Input: part model. Units: mm. Frame: model coordinates. A direction names the side the tool comes from. Give positions to 0.01 mm unless a question says otherwise; leave off trailing zeros. Use a Markdown table: item, result.
from build123d import *

# Parameters (mm, degrees)
SKETCH3_R           = 3.81
CUT_EXTRUDE1_DEPTH  = 51.8
SKETCH5_R           = 10.593705
SKETCH5_R_2         = 8.763
BOSS_EXTRUDE7_DEPTH = 17.78
SKETCH3_4_R         = 3.81
SKETCH3_4_R_2       = 1.62052
BOSS_EXTRUDE8_DEPTH = 6.35
CHAMFER1_SIZE       = 1.27


with BuildPart() as part:
    # Sketch2 → Revolve1 (revolve)
    with BuildSketch(Plane(origin=(0, 0, 0), x_dir=(0, 0, -1), z_dir=(1, 0, 0))):
        with BuildLine():
            Line((0, 50.8), (0, 47.192501809))
            ThreePointArc((0, 47.192501809), (7.113867191, 24.099005122), (8.89, 0))
            Line((8.89, 0), (19.05, 0))
            Line((19.05, 0), (19.05, 3.81))
            ThreePointArc((19.05, 3.81), (15.061820516, 27.735389015), (3.528565936, 49.073473604))
            ThreePointArc((3.528565936, 49.073473604), (1.964158278, 50.345229375), (0, 50.8))
        make_face()
    revolve(axis=Axis((0, 0, 0), (0, 1, 0)))

    # Sketch3 → Cut-Extrude1 (cut, through all)
    with BuildSketch(Plane.XZ):
        with Locations((15.11808, 0)):
            Circle(SKETCH3_R)
        with Locations((0, -15.11808)):
            Circle(SKETCH3_R)
        with Locations((-15.11808, 0)):
            Circle(SKETCH3_R)
        with Locations((0, 15.11808)):
            Circle(SKETCH3_R)
    extrude(amount=-CUT_EXTRUDE1_DEPTH, mode=Mode.SUBTRACT)

    # Sketch5 → Boss-Extrude7 (add)
    with BuildSketch(Plane(origin=(0, 6.35, 0), x_dir=(-1, 0, 0), z_dir=(0, -1, 0))):
        Circle(SKETCH5_R)
        Circle(SKETCH5_R_2, mode=Mode.SUBTRACT)
    extrude(amount=BOSS_EXTRUDE7_DEPTH)

    # Sketch3_4 → Boss-Extrude8 (add)
    with BuildSketch(Plane.XZ):
        with Locations((15.11808, 0)):
            Circle(SKETCH3_4_R)
        with Locations((15.11808, 0)):
            Circle(SKETCH3_4_R_2, mode=Mode.SUBTRACT)
        with Locations((0, -15.11808)):
            Circle(SKETCH3_4_R)
        with Locations((0, -15.11808)):
            Circle(SKETCH3_4_R_2, mode=Mode.SUBTRACT)
        with Locations((-15.11808, 0)):
            Circle(SKETCH3_4_R)
        with Locations((-15.11808, 0)):
            Circle(SKETCH3_4_R_2, mode=Mode.SUBTRACT)
        with Locations((0, 15.11808)):
            Circle(SKETCH3_4_R)
        with Locations((0, 15.11808)):
            Circle(SKETCH3_4_R_2, mode=Mode.SUBTRACT)
    extrude(amount=-BOSS_EXTRUDE8_DEPTH)

    # Chamfer1
    chamfer1_edges = [part.edges().sort_by_distance(p)[0] for p in [
        (10.593705, -11.43, 0),
    ]]
    chamfer(chamfer1_edges, length=CHAMFER1_SIZE)


solid = part.part
1. Mould query, pull axis Z, two halves, no side actions, for faces 1 (the face through (-8.36, -2.42, -2.63)), 2 (the face through (1.4, -5, -10.5)), 3 (the face through (8, 0, -8)). Classes: pulls with the +Z half, pulls with the -Z half, needs draft (parallel to the pull), parting line crosses it, or undercut.
Response:
| item | result |
|---|---|
| face 1 | undercut |
| face 2 | parting line crosses it |
| face 3 | needs draft |
2. Set-up query: faces 4 (the face through (-0.5, 17.94, -11.34)), 5 (the face through (-16.737, 3.131, 0.071)). Return all of +Z, -Z, +X, -X, +Y, -Y with unobstructed straight access to the full face (end or side cutting, diameter ignored); none if empty.
Response:
| item | result |
|---|---|
| face 4 | +Y |
| face 5 | +Y, -Y |
3. Pin query (flat end, axial travel): pin 1 (9 mm diameter, centred on x = 15.12, z = 0, fed in from +Y); pin 2 (1 mm diameter, centred on x = -2, y = 40, fed in from +Z); pin 3 (4 mm diameter, centred on y = 38, z = 6, fed in from +X); pin 4 (12 mm diameter, centred on x = 0, z = -15.12, fed in from -Y). Return the tip coordinate at first contact, or that it passes through.
Response:
| item | result |
|---|---|
| pin 1 | stops at y = 38.05 |
| pin 2 | stops at z = 9.65 |
| pin 3 | stops at x = 10.41 |
| pin 4 | stops at y = -11.43 |
4. Material intervals for line 1 along Z through (x, y) = (0, 4.75); line 2 along Z through (x, y) = (0, -2); line 3 along X through (y, z) = (0.5, 0.5), sorted ascending.
Response:
| item | result |
|---|---|
| line 1 | z = -19.04 to -16.74, -13.5 to -8.76, 8.76 to 13.5, 16.74 to 19.04 |
| line 2 | z = -10.59 to -8.76, 8.76 to 10.59 |
| line 3 | x = -19.04 to -16.66, -13.58 to -8.75, 8.75 to 13.58, 16.66 to 19.04 |
